Read the model definition and answer for the solid it produces. Units are mm, in the model's axes. Face numbers are marked on the shaded views. A direction names the side the tool comes from. Give positions to 0.01 mm unless a question says otherwise; leave off trailing zeros. Order: outer loops, then holes, each group sorted by start corner. A loop starts at its lowest first (then second) coordinate and runs counter-clockwise, first axis right, second up. Notation, with made-up numbers: (7, -8.75) -> (11, -8.75) arc R19 cw to (11, -2.75) -> close; hole circle Ø9 at (75, 65). An arc over 180 degrees is marked (long way). Answer as CSV lines item,"result". Start each with the question number.
1) Straight lines are drawn through the part: L1, parallel to X at y = 16, z = 0; L2, parallel to X at y = 40, z = 0; L3, parallel to X at y = 6.5, z = 6.5. For each, find the intervals that lie inside material, in ascending order. Write a range as from..to.
2) Find section C-C (y = 7). Determine the outline of the cut face in (x, z), and give its area (3 significant figures).
3) Find section B-B (x = 0). Determine the outline of the cut face in (y, z).
4) Find section D-D (z = 23.5). Determine the outline of the cut face in (x, y), and give its area (3 significant figures).
5) Find section A-A (z = 0). State how many separate pieces and enclosed holes the cut face has, and give its area (3 significant figures).
6) Flat-ended cylindrical pins translate along their axes: pin 1 Ø4 at (x, y) = (-32, 6) entering from +Z; pin 2 Ø20.5 at (x, z) = (63.5, -2.5) entering from +Y; pin 3 Ø4 at (y, z) = (39.5, -19) entering from -X. Find the tip coordinate at first contact, or state that the pin passes through.
7) The mould has two halves that part along X. Classify the marked faces 3, 4 and 5: +X half, -X half, draft (parallel to the pull), parting line (faces both ways), or undercut.
8) For the marked faces 1 and 2, determine the directions among +Z, -Z, +X, -X, +Y, -Y from which every point of the face is accessible in a straight line to the end or side of a thin tool.
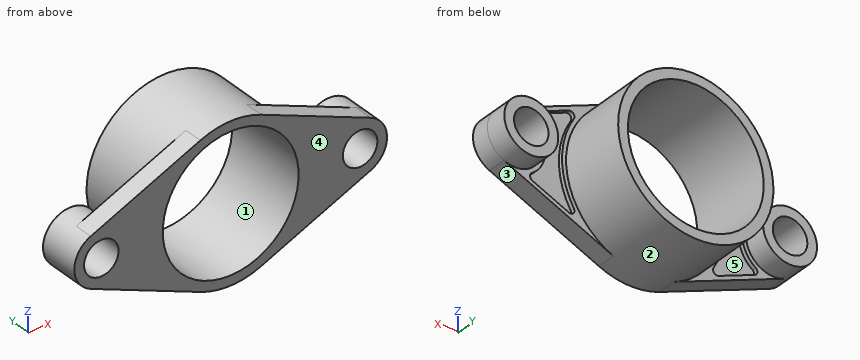
```python
from build123d import *

# Parameters (mm, degrees)
SKETCH1_R           = 10.666666667
SKETCH1_R_2         = 42
BOSS_EXTRUDE1_DEPTH = 11.5
SKETCH1_3_R         = 16.666666667
SKETCH1_3_R_2       = 10.666666667
BOSS_EXTRUDE2_DEPTH = 25
SKETCH1_4_R         = 48
SKETCH1_4_R_2       = 42
BOSS_EXTRUDE3_DEPTH = 53
CUT_EXTRUDE1_DEPTH  = 2.5


with BuildPart() as part:
    # Sketch1 → Boss-Extrude1 (new body)
    with BuildSketch(Plane(origin=(0, 0, 0), x_dir=(1, 0, 0), z_dir=(0, 1, 0))):
        with BuildLine():
            Line((-18.8, 44.165144628), (-86.527777778, 15.335119662))
            ThreePointArc((-86.527777778, 15.335119662), (-96.666666667, 0), (-86.527777778, -15.335119662))
            Line((-86.527777778, -15.335119662), (-18.8, -44.165144628))
            ThreePointArc((-18.8, -44.165144628), (0, -48), (18.8, -44.165144628))
            Line((18.8, -44.165144628), (86.527777778, -15.335119662))
            ThreePointArc((86.527777778, -15.335119662), (96.666666667, 0), (86.527777778, 15.335119662))
            Line((86.527777778, 15.335119662), (18.8, 44.165144628))
            ThreePointArc((18.8, 44.165144628), (0, 48), (-18.8, 44.165144628))
        make_face()
        with Locations(Location((-80, 0, 0), (0, 0, 270))):
            Circle(SKETCH1_R, mode=Mode.SUBTRACT)
        with Locations(Location((0, 0, 0), (0, 0, 270))):
            Circle(SKETCH1_R_2, mode=Mode.SUBTRACT)
        with Locations(Location((80, 0, 0), (0, 0, 270))):
            Circle(SKETCH1_R, mode=Mode.SUBTRACT)
    extrude(amount=BOSS_EXTRUDE1_DEPTH)

    # Sketch1_3 → Boss-Extrude2 (add)
    # profile 1 of 2: a face of its own
    with BuildSketch(Plane(origin=(0, 0, 0), x_dir=(1, 0, 0), z_dir=(0, 1, 0))):
        with Locations(Location((-80, 0, 0), (0, 0, 113.058244088))):
            Circle(SKETCH1_3_R)
        with Locations(Location((-80, 0, 0), (0, 0, 270))):
            Circle(SKETCH1_3_R_2, mode=Mode.SUBTRACT)
    # profile 2 of 2: a face of its own
    with BuildSketch(Plane(origin=(0, 0, 0), x_dir=(1, 0, 0), z_dir=(0, 1, 0))):
        with Locations(Location((80, 0, 0), (0, 0, 66.941755912))):
            Circle(SKETCH1_3_R)
        with Locations(Location((80, 0, 0), (0, 0, 270))):
            Circle(SKETCH1_3_R_2, mode=Mode.SUBTRACT)
    extrude(amount=BOSS_EXTRUDE2_DEPTH)

    # Sketch1_4 → Boss-Extrude3 (add)
    with BuildSketch(Plane(origin=(0, 0, 0), x_dir=(1, 0, 0), z_dir=(0, 1, 0))):
        with Locations(Location((0, 0, 0), (0, 0, 66.941755912))):
            Circle(SKETCH1_4_R)
        with Locations(Location((0, 0, 0), (0, 0, 270))):
            Circle(SKETCH1_4_R_2, mode=Mode.SUBTRACT)
    extrude(amount=BOSS_EXTRUDE3_DEPTH)

    # Sketch2 → Cut-Extrude1 (cut)
    with BuildSketch(Plane(origin=(0, 11.5, 0), x_dir=(1, 0, 0), z_dir=(0, 1, 0))):
        with BuildLine():
            Line((-68.749829189, -20.185673992), (-46.329311604, -29.72952886))
            ThreePointArc((-46.329311604, -29.72952886), (-43.461816215, -29.067618209), (-43.210987158, -26.135427849))
            ThreePointArc((-43.210987158, -26.135427849), (-50.5, 0), (-43.210987158, 26.135427849))
            ThreePointArc((-43.210987158, 26.135427849), (-43.461816215, 29.067618209), (-46.329311604, 29.72952886))
            Line((-46.329311604, 29.72952886), (-68.749829189, 20.185673992))
            ThreePointArc((-68.749829189, 20.185673992), (-70.258507425, 18.131633045), (-69.181739923, 15.821705345))
            ThreePointArc((-69.181739923, 15.821705345), (-60.833333333, 0), (-69.181739923, -15.821705345))
            ThreePointArc((-69.181739923, -15.821705345), (-70.258507425, -18.131633045), (-68.749829189, -20.185673992))
        make_face()
    cut_extrude1 = extrude(amount=-CUT_EXTRUDE1_DEPTH, mode=Mode.SUBTRACT)

    # Mirror1: Cut-Extrude1 across plane
    add(cut_extrude1.mirror(Plane(origin=(0, 0, 0), x_dir=(0, 0, 1), z_dir=(1, 0, 0))), mode=Mode.SUBTRACT)


solid = part.part
```
Findings below:
1,L1,"-96.67..-90.67, -69.33..-63.33, -48..-42, 42..48, 63.33..69.33, 90.67..96.67"
1,L2,"-48..-42, 42..48"
1,L3,"-95.35..-88.46, -71.54..-41.49, 41.49..71.54, 88.46..95.35"
2,outline,"(-86.53, -15.34) -> (-18.8, -44.17) arc R48 ccw to (18.8, -44.17) -> (86.53, -15.34) arc R16.67 ccw to (86.53, 15.34) -> (18.8, 44.17) arc R48 ccw to (-18.8, 44.17) -> (-86.53, 15.34) arc R16.67 ccw to start; hole circle Ø21.33 at (-80, 0); hole circle Ø84 at (0, 0); hole circle Ø21.33 at (80, 0)"
2,area,"5,770 mm²"
3,outline,"(0, -48) -> (53, -48) -> (53, -42) -> (0, -42) -> close; (0, 42) -> (53, 42) -> (53, 48) -> (0, 48) -> close"
4,outline,"(-67.35, 0) -> (-34.81, 0) -> (-34.81, 53) -> (-41.85, 53) -> (-41.85, 11.5) -> (-44.7, 11.5) -> (-44.7, 9) -> (-60.96, 9) -> (-60.96, 11.5) -> (-67.35, 11.5) -> close; (34.81, 0) -> (67.35, 0) -> (67.35, 11.5) -> (60.96, 11.5) -> (60.96, 9) -> (44.7, 9) -> (44.7, 11.5) -> (41.85, 11.5) -> (41.85, 53) -> (34.81, 53) -> close"
4,area,"1,250 mm²"
5,separate pieces,"4"
5,enclosed holes,"0"
5,area,"1,540 mm²"
6,pin 1,"z = 39.4"
6,pin 2,"y = 25"
6,pin 3,"x = -44.89"
7,face 3,"+X half"
7,face 4,"draft"
7,face 5,"undercut"
8,face 1,"+Y, -Y"
8,face 2,"+Y"
